Autodesk Inventor part; units mm, degrees
ref_plane "YZ Plane" through (0, 0, 0) normal (1, 0, 0) x (0, 1, 0)
ref_plane "XZ Plane" through (0, 0, 0) normal (0, 1, 0) x (-1, 0, 0)
ref_plane "XY Plane" through (0, 0, 0) normal (0, 0, 1) x (1, 0, 0)
sketch "Sketch1" plane through (0, 0, 0) normal (0, 0, 1) x (1, 0, 0)
  arc A0 (0.6195, 16.618) -> (12.7, 0) centre (12.7, 12.7) ccw
  arc A1 (63.5, 182.0332) -> (51.4195, 173.2512) centre (63.5, 169.3332) ccw
  line L0 (0.6195, 16.618) -> (51.4195, 173.2512)
  arc A2 (114.3, 0) -> (126.3805, 16.618) centre (114.3, 12.7) ccw
  arc A3 (75.5805, 173.2512) -> (63.5, 182.0332) centre (63.5, 169.3332) ccw
  line L1 (126.3805, 16.618) -> (75.5805, 173.2512)
  line L2 (12.7, 0) -> (114.3, 0)
  line L3 (63.5, 50.8) -> (63.5, 44.45)
  circle A4 centre (63.5, 44.45) radius 38.1
  circle A5 centre (33.655, 74.295) radius 2.1082
  circle A6 centre (93.345, 74.295) radius 2.1082
  circle A7 centre (93.345, 14.605) radius 2.1082
  circle A8 centre (33.655, 14.605) radius 2.1082
  line L4 (63.5, 82.55) -> (63.5, 86.36)
  line L5 (63.5, 86.36) -> (82.55, 86.36)
  line L6 (63.5, 86.36) -> (44.45, 86.36)
  line L7 (82.55, 86.36) -> (82.55, 134.62)
  line L8 (44.45, 86.36) -> (44.45, 134.62)
  arc A9 (82.55, 134.62) -> (44.45, 134.62) centre (63.5, 134.62) ccw
  point P0 (0, 0)
  dimension "d30" = 76.2
  dimension "d7" = 25.4
  dimension "d9" = 12.7
  dimension "d10" = 12.7
  dimension "d11" = 12.7
  dimension "d14" = 101.6
  dimension "d15" = 35.938
  dimension "d16" = 72.031
  dimension "d17" = 12.7
  dimension "d18" = 169.3332
  dimension "d19" = 109.3442
  dimension "d20" = 164.6651
  dimension "d21" = 164.6651
  dimension "d29" = 6.35
  dimension "d33" = 4.2164
  dimension "d34" = 4.2164
  dimension "d35" = 4.2164
  dimension "d36" = 4.2164
  dimension "d50" = 3.81
  dimension "d51" = 19.05
  dimension "d52" = 19.05
  dimension "d53" = 48.26
  dimension "d54" = 48.26
extrude "Extrusion2" add sketch "Sketch1" along normal blind 5.08
sketch "Sketch2" plane through (0, 0, 0) normal (0, 0, -1) x (-1, 0, 0)
  line L0 (-126.3805, 16.618) -> (-75.5805, 173.2512)
  line L1 (-126.3805, 16.618) -> (-75.5805, 173.2512)
  line L2 (-51.4195, 173.2512) -> (-0.6195, 16.618)
  line L3 (-51.4195, 173.2512) -> (-0.6195, 16.618)
  line L4 (-12.7, 0) -> (-114.3, 0)
  line L5 (-114.3, 0) -> (-12.7, 0)
  arc A0 (-126.3805, 16.618) -> (-114.3, 0) centre (-114.3, 12.7) ccw
  arc A1 (-126.3805, 16.618) -> (-126.3805, 16.618) centre (-114.3, 12.7) ccw
  arc A2 (-12.7, 0) -> (-0.6195, 16.618) centre (-12.7, 12.7) ccw
  arc A3 (-12.7, 0) -> (-12.7, 0) centre (-12.7, 12.7) ccw
  arc A4 (-51.4195, 173.2512) -> (-75.5805, 173.2512) centre (-63.5, 169.3332) ccw
  arc A5 (-75.5805, 173.2512) -> (-75.5805, 173.2512) centre (-63.5, 169.3332) ccw
  arc A6 (-49.0034, 174.0348) -> (-77.9966, 174.0348) centre (-63.5, 169.3332) ccw
  arc A7 (-128.7966, 17.4016) -> (-114.3, -2.54) centre (-114.3, 12.7) ccw
  arc A8 (-12.7, -2.54) -> (1.7966, 17.4016) centre (-12.7, 12.7) ccw
  line L6 (-12.7, -2.54) -> (-114.3, -2.54)
  line L7 (-77.9966, 174.0348) -> (-128.7966, 17.4016)
  line L8 (-49.0034, 174.0348) -> (1.7966, 17.4016)
  point P0 (0, 0)
  dimension "d57" = 30.48
  dimension "d58" = 30.48
  dimension "d59" = 30.48
extrude "Extrusion3" add sketch "Sketch2" along normal blind 71.12 and the other way blind 5.08
sketch "Sketch3" plane through (0, 0, -71.12) normal (0, 0, -1) x (-1, 0, 0)
  line L0 (-12.7, -2.54) -> (-114.3, -2.54)
  line L1 (-114.3, -2.54) -> (-12.7, -2.54)
  line L2 (1.7966, 17.4016) -> (-49.0034, 174.0348)
  line L3 (1.7966, 17.4016) -> (-49.0034, 174.0348)
  line L4 (-128.7966, 17.4016) -> (-77.9966, 174.0348)
  line L5 (-77.9966, 174.0348) -> (-128.7966, 17.4016)
  arc A0 (-128.7966, 17.4016) -> (-114.3, -2.54) centre (-114.3, 12.7) ccw
  arc A1 (-128.7966, 17.4016) -> (-114.3, -2.54) centre (-114.3, 12.7) ccw
  arc A2 (-12.7, -2.54) -> (1.7966, 17.4016) centre (-12.7, 12.7) ccw
  arc A3 (-12.7, -2.54) -> (1.7966, 17.4016) centre (-12.7, 12.7) ccw
  arc A4 (-49.0034, 174.0348) -> (-77.9966, 174.0348) centre (-63.5, 169.3332) ccw
  point P0 (0, 0)
extrude "Extrusion4" add sketch "Sketch3" along normal blind 5.08
sketch "Sketch4" plane through (0, 0, -76.2) normal (0, 0, -1) x (-1, 0, 0)
  arc A0 (-49.0034, 174.0348) -> (-77.9966, 174.0348) centre (-63.5, 169.3332) ccw
  circle A1 centre (-63.5, 169.3332) radius 2.54
  arc A2 (-126.3805, 16.618) -> (-114.3, 0) centre (-114.3, 12.7) ccw
  circle A3 centre (-114.3, 12.7) radius 2.54
  arc A4 (-12.7, 0) -> (-0.6195, 16.618) centre (-12.7, 12.7) ccw
  circle A5 centre (-12.7, 12.7) radius 2.54
  point P0 (0, 0)
  dimension "d66" = 5.08
  dimension "d67" = 5.08
  dimension "d68" = 5.08
extrude "Extrusion5" cut sketch "Sketch4" against normal blind 81.28
properties part number "Nathan_New_LED_Speaker"
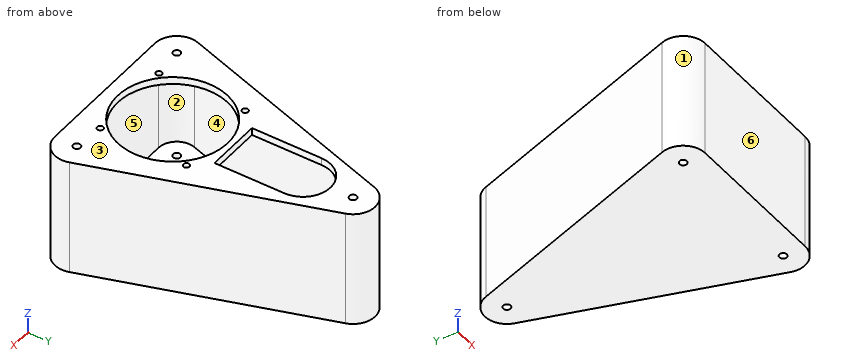
Could you check a few things on this model? Use its own coordinates, in mm. Face numbers are marked on the shaded views. A direction names the side the tool comes from. Coordinates: 2 decimals unless noted, no trailing zeros. Write each loop counter-clockwise with the first axis right and the second up, starting at its lowest first coordinate (ties: lowest second). Pieces come first, ordered by that corner, then holes. Notation, with made-up numbers: (65, -24.5) -> (85, -24.5) arc R34 cw to (85, 6.5) -> close; hole circle Ø1 at (36.25, -4.75). An arc over 180 degrees is marked (long way). Return JSON: item names as keys, results as strings.
(1) I'm going to push flat-ended pins straight in: pin 1 (6 mm diameter, centred on x = 114.3, y = 12.7, fed in from +Z); pin 2 (3.5 mm diameter, centred on x = 33.655, y = 14.605, fed in from +Z); pin 3 (5.5 mm diameter, centred on x = 72, z = 2, fed in from +Y); pin 4 (1.5 mm diameter, centred on y = 114, z = 2.5, fed in from +X). Where does each tip first touch, or does it pass through?
Numbers:
{"pin 1": "stops at z = 5.08", "pin 2": "stops at z = -71.12", "pin 3": "stops at y = 183.45", "pin 4": "stops at x = 97.71"}
(2) We'd pull the mould along Y, two halves only. Please class the marked faces 3, 4, 5 and 6: +Y half, -Y half, draft (parallel to the pull), parting line (faces both ways), or undercut.
Numbers:
{"face 3": "draft", "face 4": "undercut", "face 5": "undercut", "face 6": "-Y half"}
(3) Imagine slicing it at B-B, the plane x = 57. Please give me the cut outline in (y, z), then the cut area to 3 significant figures.
Numbers:
{"outline": "(-2.54, -76.2) -> (183.12, -76.2) -> (183.12, 5.08) -> (152.53, 5.08) -> (152.53, 0) -> (180.24, 0) -> (180.24, -71.12) -> (0, -71.12) -> (0, 0) -> (6.91, 0) -> (6.91, 5.08) -> (-2.54, 5.08) -> close; (81.99, 0) -> (86.36, 0) -> (86.36, 5.08) -> (81.99, 5.08) -> close", "area": "1,550 mm2"}
(4) Imagine slicing it at D-D, the plane x = 80.5. Please give me the cut outline in (y, z), then the cut area to 3 significant figures.
Numbers:
{"outline": "(-2.54, -76.2) -> (166.32, -76.2) -> (166.32, 5.08) -> (143.22, 5.08) -> (143.22, 0) -> (158.08, 0) -> (158.08, -71.12) -> (0, -71.12) -> (0, 0) -> (10.35, 0) -> (10.35, 5.08) -> (-2.54, 5.08) -> close; (78.55, 0) -> (86.36, 0) -> (86.36, 5.08) -> (78.55, 5.08) -> close", "area": "1,850 mm2"}
(5) Which directions (+Z, -Z, +X, -X, +Y, -Y) give clear straight access to the entire face, cutting with the end or side of a thin tool? Please do the marked faces 1 and 2.
Numbers:
{"face 1": "+Z, -Z, -X", "face 2": "none"}
(6) I need wall thicknesses on L1, parallel to Z at x = 96, y = 106.5; L2, parallel to X at y = 12, z = -72; L3, parallel to Y at x = 64.5, z = -33.5. Which ranges of each line are inside material? Lowest first, please.
Numbers:
{"L1": "z = -76.2 to -71.12, 0 to 5.08", "L2": "x = -2.52 to 10.26, 15.14 to 111.86, 116.74 to 129.52", "L3": "y = -2.54 to 0, 181.99 to 184.54"}
(7) Imagine slicing it at A-A, the plane z = -31.5. Please give me the cut outline in (x, y).
Numbers:
{"outline": "(-1.8, 17.4) arc R15.24 ccw to (12.7, -2.54) -> (114.3, -2.54) arc R15.24 ccw to (128.8, 17.4) -> (78, 174.03) arc R15.24 ccw to (49, 174.03) -> close; hole (0.62, 16.62) arc R12.7 ccw to (12.7, 0) -> (114.3, 0) arc R12.7 ccw to (126.38, 16.62) -> (75.58, 173.25) arc R12.7 ccw to (51.42, 173.25) -> close"}
(8) Imagine slicing it at C-C, the plane y = 127.5. Please give me the cut outline in (x, z), then the cut area to 3 significant figures.
Numbers:
{"outline": "(33.91, -76.2) -> (93.09, -76.2) -> (93.09, 5.08) -> (82.55, 5.08) -> (82.55, 0) -> (90.42, 0) -> (90.42, -71.12) -> (36.58, -71.12) -> (36.58, 0) -> (44.45, 0) -> (44.45, 5.08) -> (33.91, 5.08) -> close", "area": "788 mm2"}
